Design review of the part built by this model. Coordinates are the model's own, in mm. A direction names the side the tool comes from. Coordinates: 2 decimals unless noted, no trailing zeros. Order: outer loops, then holes, each group sorted by start corner. A loop starts at its lowest first (then second) coordinate and runs counter-clockwise, first axis right, second up. Notation, with made-up numbers: (9, 53) -> (21, 53) arc R37 cw to (21, 90) -> close; hole circle Ø3 at (83, 88). An arc over 180 degrees is marked (long way). Use a Markdown table: item, result. Add a question column.
Q1. Machinability: for faces 1 (the face through (0, 0, -5)), 2 (the face through (0, -11, 5)), 3 (the face through (0, 7, -0.75)), 4 (the face through (-3.64, -0.1, 5.14)), which of the approach directions +Z, -Z, +X, -X, +Y, -Y give a long, thin tool a straight path to every point of the face, cutting with its end or side? Answer none if there is none.
Q2. The part is to be moulded in two halves that separate along X. For faces 5 (the face through (-4, 0, -6)), 6 (the face through (-1.03, -7.65, 2.9)), 7 (the face through (0, 0, 5)), say which applies: pulls with the +X half, pulls with the -X half, needs draft (parallel to the pull), parting line crosses it, or undercut.
Q3. Add section C-C (x = 2.25). State the section outline as (y, z) points, then the cut area to 3 significant figures.
Q4. Wall thickness on probe 1 along Z at (x, y) = (1, 0); probe 2 along X at (y, z) = (-9, -7.5); probe 3 along Z at (x, y) = (-3.5, 1.25): over which ranges is each line inside the solid? List them lowest first.
Q5. Add section B-B (z = -10). Count the separate pieces of the cut face and the enclosed holes in it, then the cut area to 3 significant figures.
Q6. Add section A-A (x = 0). State the section outline as (y, z) points, then the cut area to 3 significant figures.
Q7. Insertion check: pin 1 (4 mm diameter, centred on x = 2, y = -10.5, fed in from +Z); pin 2 (1 mm diameter, centred on y = -2.5, z = 3, fed in from -X); pin 3 (1 mm diameter, centred on x = 0, z = -9, fed in from -Y); pin 4 (1 mm diameter, centred on x = -2, y = -8, fed in from +Z). Each pin has a flat end and moves straight along its axis. Give the tip position at first contact, or say it passes through.
Autodesk Inventor part; units mm, degrees
ref_plane "body_screw_XY" through (0, -9, 5) normal (0, 0, 1) x (1, 0, 0)
ref_plane "body_screw_YZ" through (0, -9, 5) normal (1, 0, 0) x (0, 1, 0)
ref_plane "body_screw_ZX" through (0, -9, 5) normal (0, 1, 0) x (0, 0, 1)
sketch "Sketch_1" plane through (0, 0, 0) normal (0, 0, 1) x (1, 0, 0)
  line L0 (4, 0) -> (-4, 0)
  line L1 (-4, 14.5) -> (-4, 5.5)
  line L2 (-4, 5.5) -> (-3.5, 5)
  line L3 (-3.5, 5) -> (3.5, 5)
  line L4 (3.5, 5) -> (4, 5.5)
  line L5 (4, 5.5) -> (4, 14.5)
  line L6 (4, 14.5) -> (3.5, 15)
  line L7 (3.5, 15) -> (-3.5, 15)
  line L8 (-3.5, 15) -> (-4, 14.5)
revolve "Revolution1" add sketch "Sketch_1" angle 360 about axis through (4, 0, 0) along (1, 0, 0)
sketch "Sketch_2" plane through (0, 0, 0) normal (1, 0, 0) x (0, 1, 0)
  line L0 (-15, 0.75) -> (-15, -0.75)
  line L1 (-15, -0.75) -> (9, -0.75)
  line L2 (9, -0.75) -> (9, 0.75)
  line L3 (9, 0.75) -> (-15, 0.75)
extrude "Extrusion1" cut sketch "Sketch_2" along normal mid plane 8
sketch "Sketch_3" plane through (0, 0, 0) normal (1, 0, 0) x (0, 1, 0)
  line L0 (-9, 15) -> (-9, 0)
  line L1 (-9, 0) -> (-10.7, 0)
  line L2 (-10.7, 0) -> (-10.7, 5)
  line L3 (-10.7, 5) -> (-12, 5)
  line L4 (-12, 5) -> (-12, 15)
  line L5 (-12, 15) -> (-9, 15)
  line L6 (-9, 15) -> (-9, 0)
revolve "Revolution2" cut sketch "Sketch_3" angle 360 about axis through (0, -9, 15) along (0, 0, 1)
sketch "Sketch_4" plane through (0, 0, 0) normal (1, 0, 0) x (0, 1, 0)
  line L0 (-9, -14.25) -> (-9, -0.75)
  line L1 (-9, -0.75) -> (-7.5, -0.75)
  line L2 (-7.5, -0.75) -> (-7.7705, -1.0205)
  line L3 (-7.7705, -1.0205) -> (-7.7705, -14.25)
  line L4 (-7.7705, -14.25) -> (-9, -14.25)
  line L5 (-9, -14.25) -> (-9, -0.75)
revolve "Revolution3" cut sketch "Sketch_4" angle 360 about axis through (0, -9, -14.25) along (0, 0, -1)
thread "Thread1"
sketch "Sketch_7" plane through (0, 0, -10) normal (0, 0, 1) x (1, 0, 0)
  line L0 (4, 0) -> (-4, 0)
  line L1 (-4, 0) -> (-4, 2.5)
  line L2 (-4, 2.5) -> (-3.567, 2.067)
  line L3 (-3.567, 2.067) -> (3.567, 2.067)
  line L4 (3.567, 2.067) -> (4, 2.5)
  line L5 (4, 2.5) -> (4, 0)
  line L6 (4, 0) -> (-4, 0)
revolve "Revolution4" cut sketch "Sketch_7" angle 360 about axis through (4, 0, -10) along (1, 0, 0)
thread "Thread2"
sketch "Sketch_8" plane through (0, 0, 10) normal (0, 0, 1) x (1, 0, 0)
  line L0 (4, 0) -> (-4, 0)
  line L1 (-4, 0) -> (-4, 2.5)
  line L2 (-4, 2.5) -> (-3.567, 2.067)
  line L3 (-3.567, 2.067) -> (3.567, 2.067)
  line L4 (3.567, 2.067) -> (4, 2.5)
  line L5 (4, 2.5) -> (4, 0)
  line L6 (4, 0) -> (-4, 0)
revolve "Revolution5" cut sketch "Sketch_8" angle 360 about axis through (4, 0, 10) along (1, 0, 0)
thread "Thread3"
ref_plane "body_screw_XY" through (0, -9, 5) normal (0, 0, 1) x (1, 0, 0)
ref_plane "body_screw_YZ" through (0, -9, 5) normal (1, 0, 0) x (0, 1, 0)
ref_plane "body_screw_ZX" through (0, -9, 5) normal (0, 1, 0) x (0, 0, 1)
properties part number "SSCSW10-8b" material "鉄、鋳鉄"
Established:
| question | item | result |
|---|---|---|
| 1 | face 1 | +X, -X |
| 1 | face 2 | +Z |
| 1 | face 3 | +X, -X, -Y |
| 1 | face 4 | -X |
| 2 | face 5 | pulls with the -X half |
| 2 | face 6 | undercut |
| 2 | face 7 | needs draft |
| 3 | outline | (-14.98, -0.75) arc R15 ccw (long way) to (-7.02, 13.26) -> (-7.02, 5) -> (-10.98, 5) -> (-10.98, 10.21) arc R15 ccw to (-14.98, 0.75) -> (-4.94, 0.75) arc R5 cw to (4.94, 0.75) -> (9, 0.75) -> (9, -0.75) -> (4.94, -0.75) arc R5 cw to (-4.94, -0.75) -> close; hole circle Ø4.13 at (0, -10); hole circle Ø4.13 at (0, 10) |
| 3 | area | 553 mm^2 |
| 4 | probe 1 | -15 to -12.07, -7.93 to -5, 5 to 7.93, 12.07 to 15 |
| 4 | probe 2 | -4 to -1.23, 1.23 to 4 |
| 4 | probe 3 | -14.95 to -11.65, -8.35 to -4.84, 4.84 to 8.35, 11.65 to 14.95 |
| 5 | separate pieces | 2 |
| 5 | enclosed holes | 1 |
| 5 | area | 140 mm^2 |
| 6 | outline | (-14.98, -0.75) arc R15 ccw to (-10.23, -10.97) -> (-10.23, -1.02) -> (-10.5, -0.75) -> close; (-14.98, 0.75) -> (-10.7, 0.75) -> (-10.7, 5) -> (-12, 5) -> (-12, 9) arc R15 ccw to start; (-7.77, -12.83) arc R15 ccw (long way) to (-6, 13.75) -> (-6, 5) -> (-7.3, 5) -> (-7.3, 0.75) -> (-4.94, 0.75) arc R5 cw to (4.94, 0.75) -> (9, 0.75) -> (9, -0.75) -> (4.94, -0.75) arc R5 cw to (-4.94, -0.75) -> (-7.5, -0.75) -> (-7.77, -1.02) -> close; hole circle Ø4.13 at (0, -10); hole circle Ø4.13 at (0, 10) |
| 6 | area | 498 mm^2 |
| 7 | pin 1 | z = 12.17 |
| 7 | pin 2 | through |
| 7 | pin 3 | y = -12.36 |
| 7 | pin 4 | z = 5 |
